Work out the finished part from the listing and answer in its coordinate system (mm). Face numbers are marked on the shaded views. A direction names the side the tool comes from. Coordinates: 2 decimals unless noted, no trailing zeros. Order: outer loops, then holes, each group sorted by start corner. A loop starts at its lowest first (then second) coordinate and runs counter-clockwise, first axis right, second up. Notation, with made-up numbers: M 73,63.25 L 78,63.25 A22 ccw 78,99.25 Z; hole C 62,59.25 d5. An arc over 180 degrees is marked long. Answer in a Markdown table with one row per item. Add a question column.
Item 1: The mould has two halves that part along X. Classify the marked faces 1 and 2: released by +X, released by -X, zero draft, split by the parting line, or undercut.
Item 2: The part is cut by section B-B (z = 8.75). Write down the section's boundary in (x, y), then the cut area to 3 significant figures.
Item 3: Consider line 1 (Y direction, x = 34.75, z = 5); line 2 (Y direction, x = 47.5, z = 3.75); line 3 (X direction, y = 6, z = 0.6). Determine where each line is inside the solid, lowest interval first. Write a range as from..to.
Item 4: The part is cut by section C-C (y = 6). Write down the section's boundary in (x, z).
Item 5: Which of the six approach directions +Z, -Z, +X, -X, +Y, -Y give full straight-line access (tool end or side, diameter ignored) to the marked faces 3 and 4?
Item 6: The part is cut by section D-D (y = 11.5). Write down the section's boundary in (x, z), then the cut area to 3 significant figures.
Item 7: The part is cut by section A-A (x = 34.75). Write down the section's boundary in (y, z), then the cut area to 4 significant figures.
Item 8: Flat-ended cylindrical pins translate along their axes: pin 1 Ø6 at (x, y) = (38, 5) entering from +Z; pin 2 Ø0.8 at (x, z) = (40.5, 0.5) entering from +Y; pin 3 Ø2 at (x, z) = (45.5, 2.5) entering from -Y; pin 4 Ø3 at (y, z) = (14.5, 2.5) entering from -X. Find the tip coordinate at first contact, or state that the pin passes through.
from build123d import *

# Parameters (mm, degrees)
CYLINDER010_R     = 1
CYLINDER010_DEPTH = 10
CYLINDER016_R     = 5.5
CYLINDER016_DEPTH = 10
CYLINDER012_R     = 1.75
CYLINDER012_DEPTH = 10
CYLINDER013_R     = 1.75
CYLINDER013_DEPTH = 10
CYLINDER014_R     = 5.5
CYLINDER014_DEPTH = 10
CYLINDER015_R     = 4.5
CYLINDER015_DEPTH = 10
CYLINDER011_R     = 4.5
CYLINDER011_DEPTH = 10
BOX001_W          = 16
BOX001_H          = 9
BOX001_DEPTH      = 1


with BuildPart() as cylinder010:
    # Cylinder010 → Cylinder010 (new body)
    with BuildSketch(Plane(origin=(9, 6, 0), x_dir=(1, 0, 0), z_dir=(0, 0, 1))):
        Circle(CYLINDER010_R)
    extrude(amount=CYLINDER010_DEPTH)


with BuildPart() as cylinder016:
    # Cylinder016 → Cylinder016 (new body)
    with BuildSketch(Plane(origin=(14, 0, 0), x_dir=(1, 0, 0), z_dir=(0, 0, 1))):
        Circle(CYLINDER016_R)
    extrude(amount=CYLINDER016_DEPTH)


with BuildPart() as cylinder012:
    # Cylinder012 → Cylinder012 (new body)
    with BuildSketch(Plane(origin=(17.5, 11.5, 0), x_dir=(1, 0, 0), z_dir=(0, 0, 1))):
        Circle(CYLINDER012_R)
    extrude(amount=CYLINDER012_DEPTH)


with BuildPart() as cylinder013:
    # Cylinder013 → Cylinder013 (new body)
    with BuildSketch(Plane(origin=(4.75, 11.25, 0), x_dir=(1, 0, 0), z_dir=(0, 0, 1))):
        Circle(CYLINDER013_R)
    extrude(amount=CYLINDER013_DEPTH)


with BuildPart() as fusion003:
    # Cylinder014 → Cylinder014 (new body)
    with BuildSketch(Plane(origin=(-0.5, 0, 0), x_dir=(1, 0, 0), z_dir=(0, 0, 1))):
        Circle(CYLINDER014_R)
    extrude(amount=CYLINDER014_DEPTH)

    # Fusion003: union Cylinder010, Cylinder016, Cylinder012, Cylinder013
    add(cylinder010.part)
    add(cylinder016.part)
    add(cylinder012.part)
    add(cylinder013.part)


with BuildPart() as cylinder015:
    # Cylinder015 → Cylinder015 (new body)
    with BuildSketch(Plane(origin=(17.5, 11.5, 0), x_dir=(1, 0, 0), z_dir=(0, 0, 1))):
        Circle(CYLINDER015_R)
    extrude(amount=CYLINDER015_DEPTH)


with BuildPart() as cylinder011:
    # Cylinder011 → Cylinder011 (new body)
    with BuildSketch(Plane(origin=(4.75, 11.25, 0), x_dir=(1, 0, 0), z_dir=(0, 0, 1))):
        Circle(CYLINDER011_R)
    extrude(amount=CYLINDER011_DEPTH)


with BuildPart() as cut004_button_template:
    # Box001 → Box001 (new body)
    with BuildSketch(Plane(origin=(-0.5, 3, 0), x_dir=(1, 0, 0), z_dir=(0, 0, 1))):
        with Locations((8, 4.5)):
            Rectangle(BOX001_W, BOX001_H)
    extrude(amount=BOX001_DEPTH)

    # Fusion004: union Cylinder015, Cylinder011
    add(cylinder015.part)
    add(cylinder011.part)

    # Cut004: cut Fusion003
    add(fusion003.part, mode=Mode.SUBTRACT)


with BuildPart() as cut004_button_template_1:
    # Cut004 placement: moved
    add(cut004_button_template.part.moved(Location((30, 0, 0))))


solid = cut004_button_template_1.part
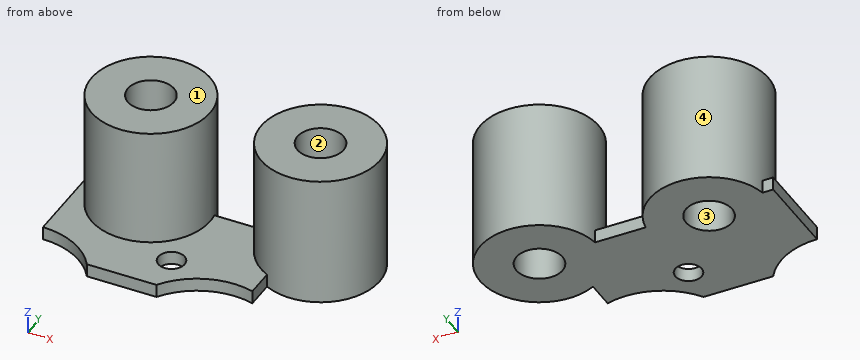
Reply:
| question | item | result |
|---|---|---|
| 1 | face 1 | zero draft |
| 1 | face 2 | undercut |
| 2 | outline | C 34.75,11.25 d9; C 47.5,11.5 d9; hole C 34.75,11.25 d3.5; hole C 47.5,11.5 d3.5 |
| 2 | area | 108 mm2 |
| 3 | line 1 | y = 6.75..9.5, 13..15.75 |
| 3 | line 2 | y = 7..9.75, 13.25..16 |
| 3 | line 3 | x = 29.5..38, 40..45.5 |
| 4 | outline | M 29.5,0 L 38,0 L 38,1 L 29.5,1 Z; M 40,0 L 45.5,0 L 45.5,1 L 40,1 Z |
| 5 | face 3 | +Z, -Z |
| 5 | face 4 | +Z |
| 6 | outline | M 29.5,0 L 33.02,0 L 33.02,10 L 30.26,10 L 30.26,1 L 29.5,1 Z; M 36.48,0 L 45.75,0 L 45.75,10 L 43,10 L 43,1 L 39.24,1 L 39.24,10 L 36.48,10 Z; M 49.25,0 L 52,0 L 52,10 L 49.25,10 Z |
| 6 | area | 115 mm2 |
| 7 | outline | M 3,0 L 9.5,0 L 9.5,10 L 6.75,10 L 6.75,1 L 3,1 Z; M 13,0 L 15.75,0 L 15.75,10 L 13,10 Z |
| 7 | area | 58.75 mm2 |
| 8 | pin 1 | stops at z = 10 |
| 8 | pin 2 | stops at y = 12 |
| 8 | pin 3 | stops at y = 7.11 |
| 8 | pin 4 | stops at x = 30.6 |
